Print and shaded views of the part. All mm, measured from the part's lowest x, y and z. Give positions to 0.01 mm unless a question says otherwise; leave off trailing zeros. Order: outer loops, then holes, each group sorted by start corner. A loop starts at its lowest first (then second) coordinate and runs counter-clockwise, first axis right, second up. Notation, with made-up numbers: (75.5, 78.25) -> (107.5, 78.25) arc R25 cw to (107.5, 116.25) -> close; hole circle Ø3 at (-28.5, 17.25). An arc over 180 degrees is marked (long way). One line per question, with ' | ' between items. Start each with the question number.
(1) Cut at B-B (y = 21.5). Give the cut face in (x, z), then the cut area to 3 significant figures.
(2) Cut at C-C (z = 6.75). Give the cut face in (x, y), then the cut area to 4 significant figures.
(3) Drill centre line: L1, parallel to X at y = 19, z = 3. Where is it in solid material? Low to high. Write a range as from..to.
(4) Pull direction Y, two halves, no side cores. Call the marked faces 1, 2 and 3: +Y half, -Y half, draft (parallel to the pull), parting line (faces both ways), or undercut.
(5) Cut at A-A (z = 11). Give the cut face in (x, y).
(6) Pin check, flat tips, straight feed: pin 1 Ø3.5 at (x, y) = (63.5, 28.5) entering from -Z; pin 2 Ø2.5 at (x, y) = (63, 28) entering from +Z; pin 3 Ø3.5 at (y, z) = (20.5, 7) entering from +X. Stop position of each tip, or through.
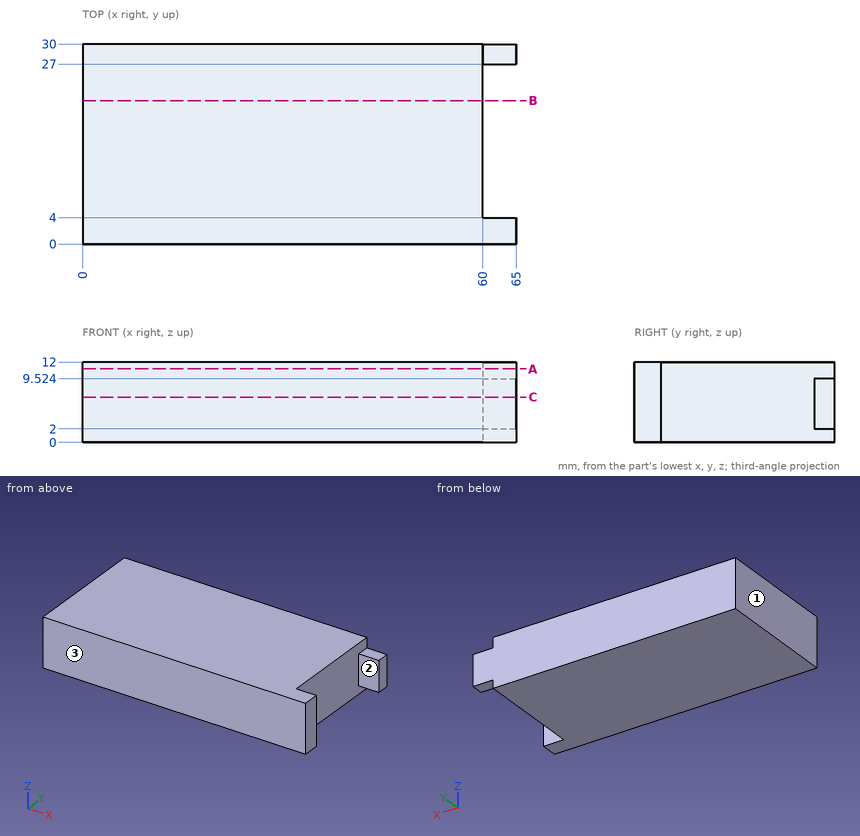
Result set:
1) outline: (0, 0) -> (60, 0) -> (60, 12) -> (0, 12) -> close | area: 720 mm2
2) outline: (0, 0) -> (65, 0) -> (65, 4) -> (60, 4) -> (60, 27) -> (65, 27) -> (65, 30) -> (0, 30) -> close | area: 1,835 mm2
3) L1: x = 0..60
4) face 1: draft | face 2: undercut | face 3: -Y half
5) outline: (0, 0) -> (65, 0) -> (65, 4) -> (60, 4) -> (60, 30) -> (0, 30) -> close
6) pin 1: stops at z = 2 | pin 2: stops at z = 9.52 | pin 3: stops at x = 60
